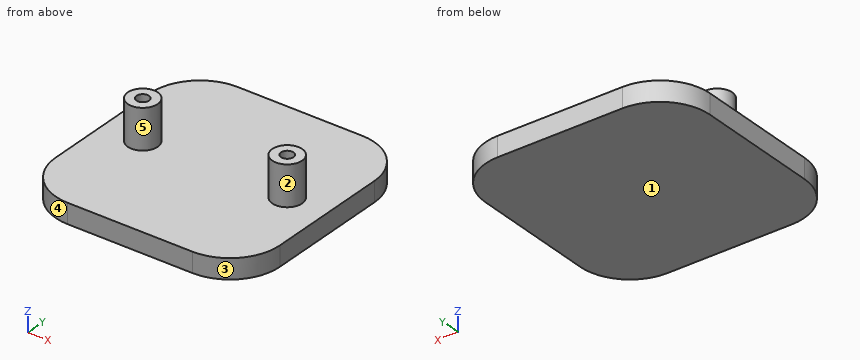
from build123d import *

# Parameters (mm, degrees)
SKETCH5_W                       = 45
SKETCH5_H                       = 45
BOSS_EXTRUDE1_DEPTH             = 4
SKETCH7_R                       = 3
BOSS_EXTRUDE2_DEPTH             = 8
SKETCH9_R                       = 3
BOSS_EXTRUDE3_DEPTH             = 8
TAP_DRILL_FOR_M3X0_5_TAP1_D     = 2.5
TAP_DRILL_FOR_M3X0_5_TAP1_DEPTH = 8
TAP_DRILL_FOR_M3X0_5_TAP1_TIP   = 0.751075774
TAP_DRILL_FOR_M3X0_5_TAP2_D     = 2.5
TAP_DRILL_FOR_M3X0_5_TAP2_DEPTH = 8
TAP_DRILL_FOR_M3X0_5_TAP2_TIP   = 0.751075774
FILLET3_R                       = 10
FILLET4_R                       = 10


with BuildPart() as part:
    # Sketch5 → Boss-Extrude1 (new body)
    with BuildSketch(Plane.XY):
        Rectangle(SKETCH5_W, SKETCH5_H)
    extrude(amount=BOSS_EXTRUDE1_DEPTH)

    # Sketch7 → Boss-Extrude2 (add)
    with BuildSketch(Plane.XY.offset(4)):
        with Locations((-14.5, 0)):
            Circle(SKETCH7_R)
    extrude(amount=BOSS_EXTRUDE2_DEPTH)

    # Sketch9 → Boss-Extrude3 (add)
    with BuildSketch(Plane.XY.offset(4)):
        with Locations((14.5, 0)):
            Circle(SKETCH9_R)
    extrude(amount=BOSS_EXTRUDE3_DEPTH)

    # Tap Drill for M3x0.5 Tap1
    with Locations(Plane.XY.offset(12)):
        with Locations((-14.5, 0)):
            Hole(TAP_DRILL_FOR_M3X0_5_TAP1_D / 2, depth=TAP_DRILL_FOR_M3X0_5_TAP1_DEPTH)
            with Locations((0, 0, -(TAP_DRILL_FOR_M3X0_5_TAP1_DEPTH + TAP_DRILL_FOR_M3X0_5_TAP1_TIP / 2))):  # 118° drill point
                Cone(0, TAP_DRILL_FOR_M3X0_5_TAP1_D / 2, TAP_DRILL_FOR_M3X0_5_TAP1_TIP, mode=Mode.SUBTRACT)

    # Tap Drill for M3x0.5 Tap2
    with Locations(Plane.XY.offset(12)):
        with Locations((14.5, 0)):
            Hole(TAP_DRILL_FOR_M3X0_5_TAP2_D / 2, depth=TAP_DRILL_FOR_M3X0_5_TAP2_DEPTH)
            with Locations((0, 0, -(TAP_DRILL_FOR_M3X0_5_TAP2_DEPTH + TAP_DRILL_FOR_M3X0_5_TAP2_TIP / 2))):  # 118° drill point
                Cone(0, TAP_DRILL_FOR_M3X0_5_TAP2_D / 2, TAP_DRILL_FOR_M3X0_5_TAP2_TIP, mode=Mode.SUBTRACT)

    # Fillet3
    fillet3_edges = [part.edges().sort_by_distance(p)[0] for p in [
        (-22.5, 22.5, 2),
    ]]
    fillet(fillet3_edges, radius=FILLET3_R)

    # Fillet4
    fillet4_edges = [part.edges().sort_by_distance(p)[0] for p in [
        (22.5, -22.5, 2),
        (-22.5, -22.5, 2),
        (22.5, 22.5, 2),
    ]]
    fillet(fillet4_edges, radius=FILLET4_R)


solid = part.part
Check sheet for the modelled part. Datum: model origin and axes. Units: mm. Face numbers are marked on the shaded views. A direction names the side the tool comes from. Round coordinates to 2 decimals unless told otherwise and drop trailing zeros. Order: outer loops, then holes, each group sorted by start corner. A loop starts at its lowest first (then second) coordinate and runs counter-clockwise, first axis right, second up.
(1) Cross-section at D-D, the plane x = 4. Enter the section's corners in (y, z), and give its area (3 significant figures).
(2) Cross-section at A-A, the plane z = 5.5. Enter the section's corners in (x, y), and give its area (3 significant figures).
(3) Access from +Z, -Z, +X, -X, +Y, -Y to the whole of each face (thin tool, end or side, straight path). Record for the marked faces 4 and 5.
(4) Cross-section at C-C, the plane y = 2. Enter the section's corners in (x, z).
(5) Go/stop test with flat-tipped pins: P1, Ø8, axis at x = 7.5, y = -1.5, coming from the +Z side; P2, Ø6, axis at y = -14.5, z = 6.5, coming from the -X side; P3, Ø4, axis at x = 10.5, z = 10.5, coming from the -Y side. Record where each tip stops, or that it passes through.
(6) Draft check along X on the marked faces 1, 2 and 3. Enter one of: pulls with the +X half, pulls with the -X half, needs draft (parallel to the pull), parting line crosses it, or undercut.
(7) Cross-section at B-B, the plane z = 1.5. Enter the section's corners in (x, y), and give its area (3 significant figures).
(8) Scan lines: probe 1 along Y at (x, z) = (14.5, 8.25); probe 2 along X at (y, z) = (-1, 7); probe 3 along Z at (x, y) = (1, -7.5). Record each from-to range of solid material in increasing order.
Check sheet entries:
1. outline: (-22.5, 0) - (22.5, 0) - (22.5, 4) - (-22.5, 4) - close
1. area: 180 mm2
2. outline: circle Ø6 at (-14.5, 0); circle Ø6 at (14.5, 0); hole circle Ø2.5 at (-14.5, 0); hole circle Ø2.5 at (14.5, 0)
2. area: 46.7 mm2
3. face 4: +Z, -Z, -X, -Y
3. face 5: +Z
4. outline: (-22.5, 0) - (22.5, 0) - (22.5, 4) - (16.74, 4) - (16.74, 12) - (12.26, 12) - (12.26, 4) - (-12.26, 4) - (-12.26, 12) - (-16.74, 12) - (-16.74, 4) - (-22.5, 4) - close
5. P1: stops at z = 4
5. P2: stops at x = -22.49
5. P3: stops at y = -2.24
6. face 1: needs draft
6. face 2: undercut
6. face 3: pulls with the +X half
7. outline: (-22.5, -12.5) arc R10 ccw to (-12.5, -22.5) - (12.5, -22.5) arc R10 ccw to (22.5, -12.5) - (22.5, 12.5) arc R10 ccw to (12.5, 22.5) - (-12.5, 22.5) arc R10 ccw to (-22.5, 12.5) - close
7. area: 1,940 mm2
8. probe 1: y = -3 to -1.25, 1.25 to 3
8. probe 2: x = -17.33 to -15.25, -13.75 to -11.67, 11.67 to 13.75, 15.25 to 17.33
8. probe 3: z = 0 to 4
